from build123d import *

# Parameters (mm, degrees)
F1_R   = 38.1
F1_R_2 = 36.449


with BuildPart() as f2:
    # F2: sweep along a path in F0
    with BuildLine(Plane.XZ) as f2_path:
        Line((-254, -63.5), (0, -63.5))
        ThreePointArc((0, -63.5), (44.901281, -44.901281), (63.5, 0))
        Line((63.5, 0), (63.5, 101.6))
    # F1 (on Right) → F2 (sweep)
    with BuildSketch(Plane.YZ):
        with Locations((0, -63.024494)):
            Circle(F1_R)
        with Locations((0, -63.024494)):
            Circle(F1_R_2, mode=Mode.SUBTRACT)
    sweep(path=f2_path.line)


solid = f2.part
Work out the finished part from the listing and answer in its coordinate system (mm). Give positions to 0.01 mm unless a question says otherwise; leave off trailing zeros. Write each loop counter-clockwise with the first axis right and the second up, starting at its lowest first coordinate (ties: lowest second). Pieces come first, ordered by that corner, then holes.
Q1. For a pull along Y with two mould halves and no side action, classify faces 1 (the face through (-254, 31, -43)), 2 (the face through (-125.222, -7.901, -98.607)), 3 (the face through (-125.22, -8.26, -100.22)) as released by +Y, released by -Y, zero draft, split by the parting line, or undercut.
Answer:
face 1: zero draft
face 2: undercut
face 3: split by the parting line
Q2. Given pin 1 (4 mm diameter, centred on y = 18, z = -43.5, fed in from -X); pin 2 (12 mm diameter, centred on y = 12, z = 58, fed in from -X); pin 3 (2 mm diameter, centred on x = -43, y = -11, fed in from +Z), each flat-ended and moving along its own axis, determine where each tip first touches the part or whether it passes through.
Answer:
pin 1: stops at x = 82.41
pin 2: stops at x = 25.4
pin 3: stops at z = -26.26
Q3. The part is cut by section A-A on x = -223.5. Give the vertices of the cut face in (y, z), and give its area (3 significant figures).
Answer:
outline: circle Ø76.2 at (0, -63.02); hole circle Ø72.9 at (0, -63.02)
area: 387 mm2
Q4. Straight lines are drawn through the part: L1, parallel to Z at x = -185, y = 0; L2, parallel to Y at x = -45, z = -56; L3, parallel to Z at x = -153.5, y = 27.5. For each, find the intervals that lie inside material, in ascending order.
Answer:
L1: z = -101.12 to -99.47, -26.58 to -24.92
L2: y = -37.45 to -35.77, 35.77 to 37.45
L3: z = -89.39 to -86.95, -39.1 to -36.65
